Verification items for the finished model (mm, model axes). A direction names the side the tool comes from. Give positions to 0.01 mm unless a question says otherwise; leave off trailing zeros. Loops run counter-clockwise (first coordinate to the right, second up) from the corner with the lowest first, then second, coordinate; pieces in that order, holes last. Notation, with made-up numbers: (-39.75, 7.25) -> (-1.75, 7.25) arc R22 ccw to (-1.75, 30.25) -> close; hole circle Ø11 at (3, 48). An arc over 180 degrees is marked (long way). Use one line per item in the form item = value. Start each with the question number.
from build123d import *

# Parameters (mm, degrees)
SKETCH1_W           = 85
SKETCH1_H           = 49
BOSS_EXTRUDE1_DEPTH = 3.175
SKETCH2_R           = 1.9
SKETCH2_R_2         = 1.4
BOSS_EXTRUDE2_DEPTH = 12.7
FILLET1_R           = 1


with BuildPart() as part:
    # Sketch1 → Boss-Extrude1 (new body)
    with BuildSketch(Plane(origin=(0, 0, 0), x_dir=(0, 0, -1), z_dir=(1, 0, 0))):
        with Locations((-11.829824561, -9.198245614)):
            Rectangle(SKETCH1_W, SKETCH1_H)
    extrude(amount=BOSS_EXTRUDE1_DEPTH)

    # Sketch2 → Boss-Extrude2 (add)
    with BuildSketch(Plane(origin=(3.175, 0, 0), x_dir=(0, 0, -1), z_dir=(1, 0, 0))):
        with Locations((-50.829824561, 11.801754386)):
            Circle(SKETCH2_R)
        with Locations((-50.829824561, 11.801754386)):
            Circle(SKETCH2_R_2, mode=Mode.SUBTRACT)
        with Locations((7.170175439, 11.801754386)):
            Circle(SKETCH2_R)
        with Locations((7.170175439, 11.801754386)):
            Circle(SKETCH2_R_2, mode=Mode.SUBTRACT)
        with Locations((7.170175439, -30.198245614)):
            Circle(SKETCH2_R)
        with Locations((7.170175439, -30.198245614)):
            Circle(SKETCH2_R_2, mode=Mode.SUBTRACT)
        with Locations((-50.829824561, -30.198245614)):
            Circle(SKETCH2_R)
        with Locations((-50.829824561, -30.198245614)):
            Circle(SKETCH2_R_2, mode=Mode.SUBTRACT)
    extrude(amount=BOSS_EXTRUDE2_DEPTH)

    # Fillet1
    fillet1_edges = [part.edges().sort_by_distance(p)[0] for p in [
        (1.5875, 15.301754386, 54.329824561),
        (1.5875, 15.301754386, -30.670175439),
        (1.5875, -33.698245614, -30.670175439),
        (1.5875, -33.698245614, 54.329824561),
    ]]
    fillet(fillet1_edges, radius=FILLET1_R)


solid = part.part
Item 1: Tool access check on faces 1 (the flat face through (3.175, -30, -7)), 2 (the flat face through (0, -9, 12)). Record the directions out of +Z, -Z, +X, -X, +Y, -Y that give a thin tool (end or side, any length) a straight path to the whole face; none if there is none.
Item 2: Gauge pin test, flat ends, axial feed: pin 1 Ø14.5 at (y, z) = (-7.5, -2) entering from +X (3 decimals); pin 2 Ø2 at (y, z) = (11.8, -7.17) entering from -X; pin 3 Ø6 at (x, y) = (7.5, 2) entering from +Z. Record the tip position at first contact, or that the pin passes through.
Item 3: Sectioned sample at C-C, the plane y = -15. Enter the section's corners in (x, z) (3 decimals), and give its area (3 significant figures).
Item 4: Material ranges on line 1 (Z direction, x = 3.5, y = -29.5); line 2 (Z direction, x = 14.25, y = 13); line 3 (X direction, y = 12, z = -1) (3 decimals), recorded low to high.
Item 5: Sectioned sample at A-A, the plane x = 12.75. Enter the section's corners in (y, z), and give its area (3 significant figures).
Item 6: Draft check along Y on faces 3 (the cylindrical face through (9.436, -29.628, 49.018)), 4 (the cylindrical face through (9.436, 12.372, 49.018)), 5 (the flat face through (2, -10, -30.67)), 6 (the flat face through (2, -33.698, 12)). Enter one of: +Y half, -Y half, draft (parallel to the pull), parting line (faces both ways), or undercut.
Item 7: Sectioned sample at B-B, the plane z = 22.5. Enter the section's corners in (x, y) (3 decimals).
Outcome:
q1.face_1 = +X
q1.face_2 = +Z, -Z, -X, +Y, -Y
q2.pin_1 = 3.175
q2.pin_2 = 0
q2.pin_3 = through
q3.outline = (0, -30.67) -> (3.175, -30.67) -> (3.175, 54.33) -> (0, 54.33) -> close
q3.area = 270 mm^2
q4.line_1 = -8.94 to -8.38, -5.96 to -5.4, 49.06 to 49.62, 52.04 to 52.6
q4.line_2 = -8.64 to -7.89, -6.45 to -5.7, 49.36 to 50.11, 51.55 to 52.3
q4.line_3 = 0 to 3.175
q5.outline = circle Ø3.8 at (-30.2, -7.17); circle Ø3.8 at (-30.2, 50.83); circle Ø3.8 at (11.8, -7.17); circle Ø3.8 at (11.8, 50.83); hole circle Ø2.8 at (-30.2, -7.17); hole circle Ø2.8 at (-30.2, 50.83); hole circle Ø2.8 at (11.8, -7.17); hole circle Ø2.8 at (11.8, 50.83)
q5.area = 20.7 mm^2
q6.face_3 = undercut
q6.face_4 = undercut
q6.face_5 = draft
q6.face_6 = -Y half
q7.outline = (0, -33.698) -> (3.175, -33.698) -> (3.175, 15.302) -> (0, 15.302) -> close
